For this review, take the finished solid that the model builds, in its own axes (mm). A direction names the side the tool comes from. Coordinates: 2 decimals unless noted, no trailing zeros. Write each loop counter-clockwise with the first axis right and the second up, starting at its lowest first coordinate (ties: lowest second). Pieces come first, ordered by that corner, then holes. Notation, with made-up numbers: M -40,49.5 L 6,49.5 A19 ccw 6,54.5 Z; hole C 4,73 d9. An arc over 180 degrees is marked long. One line per question, with ' | ' between items.
Autodesk Inventor part; units mm, degrees
ref_plane "YZ Plane" through (0, 0, 0) normal (1, 0, 0) x (0, 1, 0)
ref_plane "XZ Plane" through (0, 0, 0) normal (0, 1, 0) x (-1, 0, 0)
ref_plane "XY Plane" through (0, 0, 0) normal (0, 0, 1) x (1, 0, 0)
sketch "草圖1" plane through (0, 0, 0) normal (0, 1, 0) x (-1, 0, 0)
  line L0 (0, 0) -> (6, 0)
  line L1 (6, 0) -> (6, -24.6)
  line L2 (6, -24.6) -> (0, -24.6)
  line L3 (0, -24.6) -> (0, 0)
  line L4 (1, 0) -> (5, 0)
  line L5 (5, 0) -> (5, 3)
  line L6 (5, 3) -> (1, 3)
  line L7 (1, 3) -> (1, 0)
  line L8 (5, -24.6) -> (1, -24.6)
  line L9 (1, -24.6) -> (1, -27.6)
  line L10 (1, -27.6) -> (5, -27.6)
  line L11 (5, -27.6) -> (5, -24.6)
  line L12 (3, 0) -> (3, -24.6)
  line L13 (6, -12.3) -> (0, -12.3)
  circle A0 centre (3, -12.3) radius 1.4
  dimension "d0" = 24.6
  dimension "d1" = 6
  dimension "d2" = 4
  dimension "d3" = 3
  dimension "d4" = 3
  dimension "d5" = 4
  dimension "d6" = 2.8
extrude "擠出1" add sketch "草圖1" along normal blind 3 contours L0 L12 A0 L13 L3 | L7 L6 L5 L0 | L13 A0 L12 L2 L3 | L0 L1 L13 A0 L12 | L2 L11 L10 L9 | A0 L13 L1 L2 L12
properties part number "螺絲"
1) We need section B-B on x = -3. State the section outline as (y, z) points, then the cut area to 3 significant figures.
Responses:
outline: M 0,-27.6 L 3,-27.6 L 3,-13.7 L 0,-13.7 Z; M 0,-10.9 L 3,-10.9 L 3,3 L 0,3 Z | area: 83.4 mm^2
2) We need section A-A on y = 1.95. State the section outline as (x, z) points.
Responses:
outline: M -6,-24.6 L -5,-24.6 L -5,-27.6 L -1,-27.6 L -1,-24.6 L 0,-24.6 L 0,0 L -1,0 L -1,3 L -5,3 L -5,0 L -6,0 Z; hole C -3,-12.3 d2.8
3) We need section C-C on z = -12.3. State the section outline as (x, y) points.
Responses:
outline: M -6,0 L -4.4,0 L -4.4,3 L -6,3 Z; M -1.6,0 L 0,0 L 0,3 L -1.6,3 Z
4) The part is to be moulded in two halves that separate along Z. For faces 1 (the cylindrical face through (-2.697, 1.479, -10.933)), 2 (the flat face through (-0.5, 1.5, -24.6)), 3 (the flat face through (0, 1, -12)), say which applies: +Z half, -Z half, draft (parallel to the pull), parting line (faces both ways), or undercut.
Responses:
face 1: undercut | face 2: -Z half | face 3: draft
5) Insertion check: pin 1 Ø0.5 at (x, y) = (-5.5, 1.5) entering from +Z; pin 2 Ø2.5 at (x, z) = (-3, -12.3) entering from -Y; pin 3 Ø0.9 at (y, z) = (2, -26) entering from +X. Each pin has a flat end and moves straight along its axis. Give the tip position at first contact, or say it passes through.
Responses:
pin 1: z = 0 | pin 2: through | pin 3: x = -1
6) Machinability: for faces 4 (the flat face through (-1, 1, -26)), 5 (the flat face through (-5, 1, 1)), 6 (the flat face through (-3, 1, -27.6)), 7 (the flat face through (-0.5, 1.5, 0)), 8 (the flat face through (-5, 1, -26)), which of the approach directions +Z, -Z, +X, -X, +Y, -Y give a long, thin tool a straight path to every point of the face, cutting with its end or side? Answer none if there is none.
Responses:
face 4: -Z, +X, +Y, -Y | face 5: +Z, -X, +Y, -Y | face 6: -Z, +X, -X, +Y, -Y | face 7: +Z, +X, +Y, -Y | face 8: -Z, -X, +Y, -Y
7) To check wall thickness, follow line 1 along Z through (x, y) = (-3, 1.15); line 2 along X through (y, z) = (2, -12.3); line 3 along Z through (x, y) = (-5.15, 1.6). State the ranges of each line that lie inside material, in increasing order. Write a range as [from, to].
Responses:
line 1: [-27.6, -13.7], [-10.9, 3] | line 2: [-6, -4.4], [-1.6, 0] | line 3: [-24.6, 0]
